Source: three-view drawing plus pictorial views. Frame: mm from the lowest corner of the part. Give positions to 0.01 mm unless a question says otherwise; leave off trailing zeros. Loops run counter-clockwise (first coordinate to the right, second up) from the corner with the lowest first, then second, coordinate; pieces in that order, holes last. Notation, with made-up numbers: (-11.5, -21.5) - (6.5, -21.5) arc R35 ccw to (6.5, 12.5) - close; hole circle Ø11 at (32.5, 89). An arc over 180 degrees is marked (long way). Write each question's results on one line, items separated by ' | '. Start each with the question number.
(1) Contact query for a flat-ended pin moving along its axis: pin 1 (3 mm diameter, centred on x = 2.5, y = 2.5, fed in from +Z). Output: stop coordinate, or through.
(2) Material intervals for line 1 along X through (y, z) = (2.5, 0.4); line 2 along X through (y, z) = (3, 0.8), sorted ascending. Write a range as [from, to].
(3) Cut plane A-A on y = 2.5. Return the cut outline in (x, z).
(4) Cut plane C-C on z = 1.6. Return the cut outline in (x, y), then the cut area to 3 significant figures.
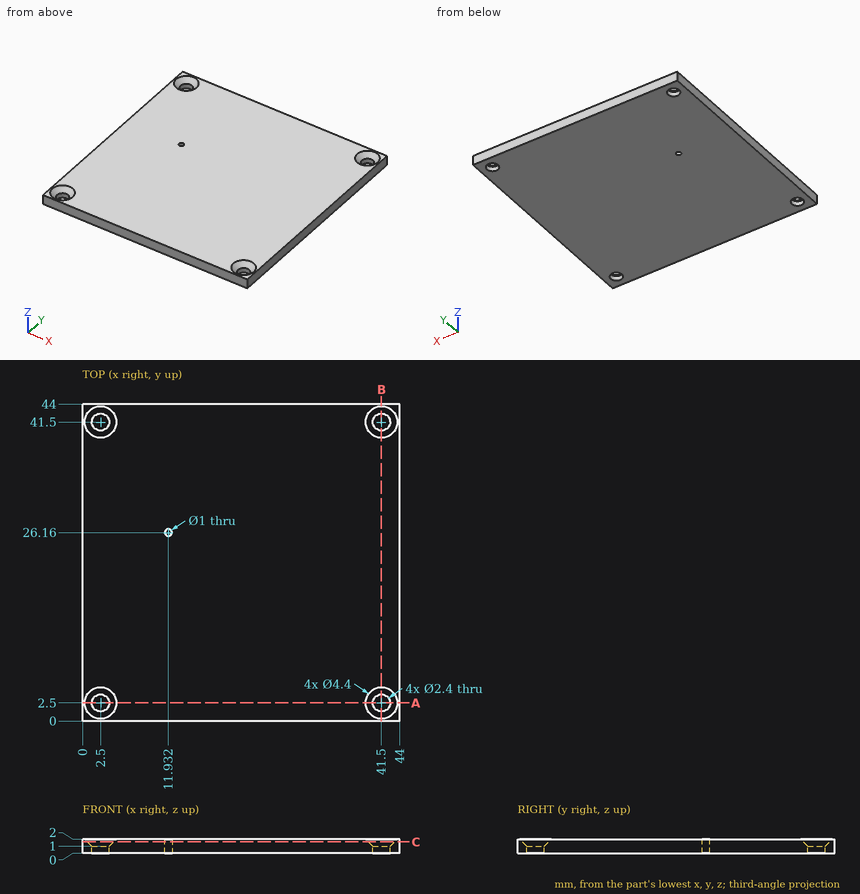
Ans:
1) pin 1: z = 1.3
2) line 1: [0, 1.3], [3.7, 40.3], [42.7, 44] | line 2: [0, 1.41], [3.59, 40.41], [42.59, 44]
3) outline: (0, 0) - (1.3, 0) - (1.3, 1) - (0.3, 2) - (0, 2) - close; (3.7, 0) - (40.3, 0) - (40.3, 1) - (39.3, 2) - (4.7, 2) - (3.7, 1) - close; (42.7, 0) - (44, 0) - (44, 2) - (43.7, 2) - (42.7, 1) - close
4) outline: (0, 0) - (44, 0) - (44, 44) - (0, 44) - close; hole circle Ø3.6 at (2.5, 2.5); hole circle Ø3.6 at (2.5, 41.5); hole circle Ø1 at (11.93, 26.16); hole circle Ø3.6 at (41.5, 2.5); hole circle Ø3.6 at (41.5, 41.5) | area: 1,890 mm^2
